Read the model definition and answer for the solid it produces. Units are mm, in the model's axes. A direction names the side the tool comes from. Give positions to 0.01 mm unless a question says otherwise; leave off trailing zeros. Order: outer loops, then holes, each group sorted by start corner. A loop starts at its lowest first (then second) coordinate and runs counter-clockwise, first axis right, second up. Notation, with made-up numbers: (43, 83.5) - (78, 83.5) arc R34 ccw to (78, 117.5) - close; hole circle Ø2 at (80, 12.5). An arc over 180 degrees is marked (long way). Return JSON: item names as keys, results as strings.
```python
from build123d import *

# Parameters (mm, degrees)
SKETCH1_W           = 1500
SKETCH1_H           = 1000
BOSS_EXTRUDE1_DEPTH = 50
SKETCH2_W           = 1000
SKETCH2_H           = 1000
BOSS_EXTRUDE2_DEPTH = 200
SKETCH3_W           = 900
SKETCH3_H           = 950
CUT_EXTRUDE1_DEPTH  = 150
SKETCH4_W           = 100
SKETCH4_H           = 50
BOSS_EXTRUDE3_DEPTH = 400
SKETCH5_W           = 50
SKETCH5_H           = 50
CUT_EXTRUDE2_DEPTH  = 110
SKETCH7_W           = 1500
SKETCH7_H           = 500
CUT_EXTRUDE3_DEPTH  = 1347.291201784
SKETCH8_W           = 1500
SKETCH8_H           = 297.02623805
CUT_EXTRUDE4_DEPTH  = 1347.291201784
SKETCH9_W           = 250
SKETCH9_H           = 202.97376195
CUT_EXTRUDE5_DEPTH  = 1267.372120682
SKETCH10_R          = 313.8
CUT_EXTRUDE6_DEPTH  = 20


with BuildPart() as part:
    # Sketch1 → Boss-Extrude1 (new body)
    with BuildSketch(Plane(origin=(0, 0, 0), x_dir=(1, 0, 0), z_dir=(0, 1, 0))):
        Rectangle(SKETCH1_W, SKETCH1_H)
    extrude(amount=BOSS_EXTRUDE1_DEPTH)

    # Sketch2 → Boss-Extrude2 (add)
    with BuildSketch(Plane.XY):
        with Locations((0, 550)):
            Rectangle(SKETCH2_W, SKETCH2_H)
    extrude(amount=-BOSS_EXTRUDE2_DEPTH)

    # Sketch3 → Cut-Extrude1 (cut)
    with BuildSketch(Plane.XY):
        with Locations((0, 525)):
            Rectangle(SKETCH3_W, SKETCH3_H)
    extrude(amount=-CUT_EXTRUDE1_DEPTH, mode=Mode.SUBTRACT)

    # Sketch4 → Boss-Extrude3 (add)
    with BuildSketch(Plane(origin=(0, 50, 0), x_dir=(1, 0, 0), z_dir=(0, 1, 0))):
        with Locations((0, 25)):
            Rectangle(SKETCH4_W, SKETCH4_H)
    extrude(amount=BOSS_EXTRUDE3_DEPTH)

    # Sketch5 → Cut-Extrude2 (cut)
    with BuildSketch(Plane(origin=(500, 0, 0), x_dir=(0, 0, -1), z_dir=(1, 0, 0))):
        with Locations((70, 525)):
            Rectangle(SKETCH5_W, SKETCH5_H)
    extrude(amount=-CUT_EXTRUDE2_DEPTH, mode=Mode.SUBTRACT)

    # Sketch7 → Cut-Extrude3 (cut, through all)
    with BuildSketch(Plane(origin=(0, 50, 0), x_dir=(1, 0, 0), z_dir=(0, 1, 0))):
        with Locations((0, -250)):
            Rectangle(SKETCH7_W, SKETCH7_H)
    extrude(amount=-CUT_EXTRUDE3_DEPTH, mode=Mode.SUBTRACT)

    # Sketch8 → Cut-Extrude4 (cut, through all)
    with BuildSketch(Plane(origin=(0, 50, 0), x_dir=(1, 0, 0), z_dir=(0, 1, 0))):
        with Locations((0, 351.486880975)):
            Rectangle(SKETCH8_W, SKETCH8_H)
    extrude(amount=-CUT_EXTRUDE4_DEPTH, mode=Mode.SUBTRACT)

    # Sketch9 → Cut-Extrude5 (cut, through all)
    with BuildSketch(Plane(origin=(0, 50, 0), x_dir=(1, 0, 0), z_dir=(0, 1, 0))):
        with Locations((-625, 101.486880975)):
            Rectangle(SKETCH9_W, SKETCH9_H)
        with Locations((625, 101.486880975)):
            Rectangle(SKETCH9_W, SKETCH9_H)
    extrude(amount=-CUT_EXTRUDE5_DEPTH, mode=Mode.SUBTRACT)

    # Sketch10 → Cut-Extrude6 (cut)
    with BuildSketch(Plane.XY.offset(-150)):
        with Locations((0, 530)):
            Circle(SKETCH10_R)
    extrude(amount=-CUT_EXTRUDE6_DEPTH, mode=Mode.SUBTRACT)


solid = part.part
```
Q1. A cutting plane is placed at D-D (y = 882). Write down the section's boundary in (x, z).
Values:
{"outline": "(-500, -200) - (500, -200) - (500, 0) - (450, 0) - (450, -150) - (-450, -150) - (-450, 0) - (-500, 0) - close"}
Q2. Consider L1, parallel to Y at x = 76, z = -72.5; L2, parallel to Y at x = 0, z = -156; L3, parallel to X at y = 286.5, z = -61.5. Determine where each line is inside the solid, lowest interval first.
Values:
{"L1": "y = 0 to 50, 1000 to 1050", "L2": "y = 0 to 216.2, 843.8 to 1050", "L3": "x = -500 to -450, 450 to 500"}
Q3. Given pin 1 (1.5 mm diameter, centred on x = -212.5, y = 767, fed in from -Z); pin 2 (0.9 mm diameter, centred on x = 15.5, z = -201.5, fed in from +Y), each flat-ended and moving along its own axis, determine where each tip first touches the part or whether it passes through.
Values:
{"pin 1": "stops at z = -200", "pin 2": "stops at y = 50"}
Q4. A cutting plane is placed at B-B (y = 99.5). Write down the section's boundary in (x, z).
Values:
{"outline": "(-500, -200) - (500, -200) - (500, 0) - (450, 0) - (450, -150) - (-450, -150) - (-450, 0) - (-500, 0) - close; (-50, -50) - (50, -50) - (50, 0) - (-50, 0) - close"}
Q5. For faces 1 (the flat face through (-50, 247, -25)), 2 (the flat face through (-7, 557, -200)), 3 (the flat face through (475, 550, -70)), 4 (the flat face through (-7, 25, -202.974)), determine the directions among +Z, -Z, +X, -X, +Y, -Y from which every point of the face is accessible in a straight line to the end or side of a thin tool.
Values:
{"face 1": "+Z", "face 2": "-Z, +X, -X, +Y", "face 3": "+X", "face 4": "-Z, +X, -X, +Y, -Y"}
Q6. A cutting plane is placed at C-C (x = 393). Write down the section's boundary in (y, z), and give its area (3 significant figures).
Values:
{"outline": "(0, -202.97) - (50, -202.97) - (50, -200) - (1050, -200) - (1050, 0) - (1000, 0) - (1000, -150) - (50, -150) - (50, 0) - (0, 0) - close", "area": "67,600 mm²"}
Q7. Determine the mould class of faces 5 (the flat face through (475, 500, -70)), 6 (the flat face through (450, 518, -107)), 7 (the flat face through (-500, 532, -100)), 8 (the flat face through (500, 532, -100)) for opening direction X: released by +X, released by -X, zero draft, split by the parting line, or undercut.
Values:
{"face 5": "zero draft", "face 6": "undercut", "face 7": "released by -X", "face 8": "released by +X"}
Q8. A cutting plane is placed at A-A (z = -24). Write down the section's boundary in (x, y), and give its area (3 significant figures).
Values:
{"outline": "(-500, 0) - (500, 0) - (500, 1050) - (-500, 1050) - close; hole (-450, 50) - (-50, 50) - (-50, 450) - (50, 450) - (50, 50) - (450, 50) - (450, 1000) - (-450, 1000) - close", "area": "235,000 mm²"}
